from build123d import *

# Parameters (mm, degrees)
BOSS_EXTRUDE1_DEPTH = 250
BOSS_EXTRUDE2_DEPTH = 250
FILLET1_R           = 0.75
FILLET2_R           = 1.25


with BuildPart() as part:
    # Sketch3 → Boss-Extrude1 (new, symmetric)
    with BuildSketch(Plane.XY):
        with BuildLine():
            Line((12.5, -10), (17.9, -10))
            ThreePointArc((17.9, -10), (19.38492424, -9.38492424), (20, -7.9))
            Line((20, -7.9), (20, -2.5))
            Line((20, -2.5), (18.213351365, -2.5))
            Line((18.213351365, -2.5), (18.213351365, -6.95))
            Line((18.213351365, -6.95), (13.6, -2.336648635))
            Line((13.6, -2.336648635), (13.6, 0))
            Line((13.6, 0), (12.15, 0))
            ThreePointArc((12.15, 0), (11.52027958, -1.52027958), (10, -2.15))
            Line((10, -2.15), (10, -3.6))
            Line((10, -3.6), (12.336648635, -3.6))
            Line((12.336648635, -3.6), (16.95, -8.213351365))
            Line((16.95, -8.213351365), (12.5, -8.213351365))
            Line((12.5, -8.213351365), (12.5, -10))
        make_face()
    extrude(amount=BOSS_EXTRUDE1_DEPTH, both=True)

    # Sketch4 → Boss-Extrude2 (add, symmetric)
    with BuildSketch(Plane.XY):
        with BuildLine():
            Line((10, -3.6), (7.663351365, -3.6))
            Line((7.663351365, -3.6), (3.05, -8.213351365))
            Line((3.05, -8.213351365), (7.5, -8.213351365))
            Line((7.5, -8.213351365), (7.5, -10))
            Line((7.5, -10), (0, -10))
            Line((0, -10), (0, -8.736648635))
            Line((0, -8.736648635), (6.4, -2.336648635))
            Line((6.4, -2.336648635), (6.4, 0))
            Line((6.4, 0), (7.85, 0))
            ThreePointArc((7.85, 0), (8.47972042, -1.52027958), (10, -2.15))
            Line((10, -2.15), (10, -3.6))
        make_face()
    extrude(amount=BOSS_EXTRUDE2_DEPTH, both=True)

    # Mirror1: part across plane


with BuildPart() as part_1:
    add(part.part)
    add(part.part.mirror(Plane(origin=(0, 0, 0), x_dir=(0, 0, 1), z_dir=(1, 0, 0))))

    # Mirror2: part across plane


with BuildPart() as part_2:
    add(part_1.part)
    add(part_1.part.mirror(Plane.ZX))

    # Fillet1
    fillet1_edges = [part_2.edges().sort_by_distance(p)[0] for p in [
        (18.213351365, 6.95, 0),
        (13.6, 2.336648635, 0),
        (12.336648635, 3.6, 0),
        (16.95, 8.213351365, 0),
        (3.05, 8.213351365, 0),
        (7.663351365, 3.6, 0),
        (-18.213351365, 6.95, 0),
        (-13.6, 2.336648635, 0),
        (-7.663351365, 3.6, 0),
        (-12.336648635, 3.6, 0),
        (-16.95, 8.213351365, 0),
        (-3.05, 8.213351365, 0),
        (16.95, -8.213351365, 0),
        (12.336648635, -3.6, 0),
        (13.6, -2.336648635, 0),
        (18.213351365, -6.95, 0),
        (3.05, -8.213351365, 0),
        (7.663351365, -3.6, 0),
        (-18.213351365, -6.95, 0),
        (-13.6, -2.336648635, 0),
        (-12.336648635, -3.6, 0),
        (-16.95, -8.213351365, 0),
        (-3.05, -8.213351365, 0),
        (-7.663351365, -3.6, 0),
    ]]
    fillet(fillet1_edges, radius=FILLET1_R)

    # Fillet2
    fillet2_edges = [part_2.edges().sort_by_distance(p)[0] for p in [
        (6.4, 2.336648635, 0),
        (0, 8.736648635, 0),
        (-6.4, 2.336648635, 0),
        (6.4, -2.336648635, 0),
        (-6.4, -2.336648635, 0),
        (0, -8.736648635, 0),
    ]]
    fillet(fillet2_edges, radius=FILLET2_R)


solid = part_2.part
Input: part model. Units: mm. Frame: model coordinates. Coordinates: 2 decimals unless noted, no trailing zeros. Answer in a Markdown table with one row per item.
(1) Section query A-A, the plane z = 209. Give the number of separate pieces and of enclosed holes in the cut face, plus the area to 3 significant figures.
Numbers:
| item | result |
|---|---|
| separate pieces | 1 |
| enclosed holes | 3 |
| area | 324 mm^2 |
(2) Contact query for flat-ended pins moving along their axis: pin 1 Ø2 at (x, z) = (10.5, -74.5) entering from -Y; pin 2 Ø0.5 at (y, z) = (-9.5, -32.5) entering from +X; pin 3 Ø2 at (y, z) = (9, -101.5) entering from +X. Output: stop coordinate, or through.
Numbers:
| item | result |
|---|---|
| pin 1 | stops at y = -3.6 |
| pin 2 | stops at x = 19.51 |
| pin 3 | stops at x = 20 |
(3) Material intervals for line 1 (X direction, y = 0, z = -36); line 2 (Y direction, x = -6.5, z = -104); line 3 (Y direction, x = 4.5, z = -107), sorted ascending. Write a range as [from, to].
Numbers:
| item | result |
|---|---|
| line 1 | x = [-13.6, -12.15], [-7.85, -6.4], [6.4, 7.85], [12.15, 13.6] |
| line 2 | y = [-10, -8.21], [-4.76, 4.76], [8.21, 10] |
| line 3 | y = [-10, -8.12], [-6.76, -4.24], [4.24, 6.76], [8.12, 10] |
